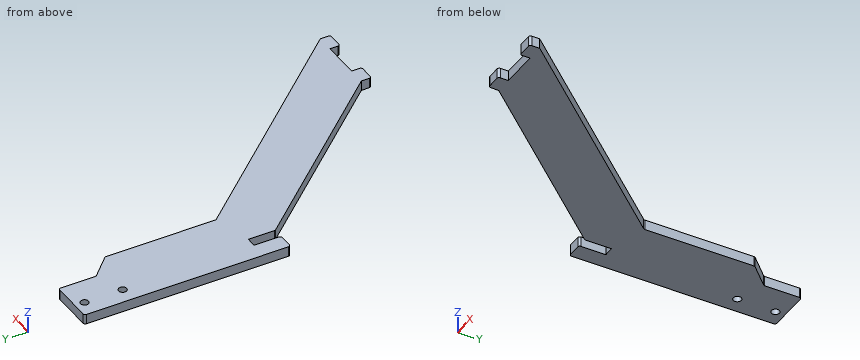
```python
from build123d import *

# Parameters (mm, degrees)
SKETCH1_R           = 1.89865
BOSS_EXTRUDE1_DEPTH = 4.7625


with BuildPart() as part:
    # Sketch1 → Boss-Extrude1 (new body)
    with BuildSketch(Plane.XY):
        with BuildLine():
            Line((-2.175, 27), (17.118365096, 27))
            ThreePointArc((17.118365096, 27), (17.825471878, 26.707106781), (18.118365096, 26))
            Line((18.118365096, 26), (18.118365096, 9.664213562))
            ThreePointArc((18.118365096, 9.664213562), (18.194485564, 9.28153013), (18.411258315, 8.957106781))
            Line((18.411258315, 8.957106781), (27.707106781, -0.338741685))
            ThreePointArc((27.707106781, -0.338741685), (27.923879533, -0.663165034), (28, -1.045848466))
            Line((28, -1.045848466), (28, -52.620004972))
            ThreePointArc((28, -52.620004972), (28.065214876, -52.975218671), (28.252353545, -53.284101936))
            Line((28.252353545, -53.284101936), (116.825, -153))
            Line((116.825, -153), (116.825, -156.7625))
            ThreePointArc((116.825, -156.7625), (116.532106781, -157.469606781), (115.825, -157.7625))
            Line((115.825, -157.7625), (109.825, -157.7625))
            ThreePointArc((109.825, -157.7625), (109.117893219, -157.469606781), (108.825, -156.7625))
            Line((108.825, -156.7625), (108.825, -153))
            Line((108.825, -153), (90.851723172, -153))
            Line((90.851723172, -153), (90.851723172, -156.7625))
            ThreePointArc((90.851723172, -156.7625), (90.558829954, -157.469606781), (89.851723172, -157.7625))
            Line((89.851723172, -157.7625), (83.851723172, -157.7625))
            ThreePointArc((83.851723172, -157.7625), (83.144616391, -157.469606781), (82.851723172, -156.7625))
            Line((82.851723172, -156.7625), (82.851723172, -153))
            Line((82.851723172, -153), (9.777353545, -70.73220419))
            ThreePointArc((9.777353545, -70.73220419), (9.590214876, -70.423320926), (9.525, -70.068107226))
            Line((9.525, -70.068107226), (9.525, -57.748102255))
            Line((9.525, -57.748102255), (4.7625, -57.748102255))
            Line((4.7625, -57.748102255), (4.7625, -69.448102255))
            ThreePointArc((4.7625, -69.448102255), (4.469606781, -70.155209036), (3.7625, -70.448102255))
            Line((3.7625, -70.448102255), (-2.175, -70.448102255))
            ThreePointArc((-2.175, -70.448102255), (-2.882106781, -70.155209036), (-3.175, -69.448102255))
            Line((-3.175, -69.448102255), (-3.175, 26))
            ThreePointArc((-3.175, 26), (-2.882106781, 26.707106781), (-2.175, 27))
        make_face()
        with Locations(Location((4.5, 22.5, 0), (0, 0, 180))):
            Circle(SKETCH1_R, mode=Mode.SUBTRACT)
        with Locations(Location((4.5, 4.5, 0), (0, 0, 180))):
            Circle(SKETCH1_R, mode=Mode.SUBTRACT)
    extrude(amount=BOSS_EXTRUDE1_DEPTH)


solid = part.part
```
Can you work these out from the model? Positions are in its coordinate system, mm. Give positions to 0.01 mm unless a question says otherwise; leave off trailing zeros. Loops run counter-clockwise (first coordinate to the right, second up) from the corner with the lowest first, then second, coordinate; pieces in that order, holes last. Notation, with made-up numbers: M -4.5,-13.75 L 39.5,-13.75 A34 ccw 39.5,20.25 Z; hole C 28.25,25 d7. An arc over 180 degrees is marked long. Use CSV: the item, a comma, the result in double quotes. Start each with the question number.
1. For P1, Ø2.5, axis at x = 103.5, z = 3, coming from the -Y side; P2, Ø1.1, axis at y = -155.5, z = 3, coming from the -X side; P3, Ø2.5, axis at y = 19, z = 3, coming from the +X side, each with a flat end and sliding along its axis, tell me the tip position at first contact or that it passes through.
2. Imagine slicing it at A-A, the plane y = 22.5. Write out the boundary of the cut face in (x, z) (1 decimal).
3. If I drill on L1, parallel to Y at x = 4.5, z = 1.25; L2, parallel to X at y = 22.5, z = 2.85 (3 decimals); L3, parallel to X at y = -1, z = 1.95 (3 decimals), over which ranges is the centre line in solid material (lowest first)?
4. Imagine slicing it at C-C, the plane y = -28.5. Write out the boundary of the cut face in (x, z) (1 decimal), plus the area to 3 significant figures.
5. Imagine slicing it at B-B, the plane z = 1.95. Count the separate pieces of the cut face and the enclosed holes in it, plus the area to 3 significant figures.
6. Imagine slicing it at D-D, the plane x = 45. Write out the boundary of the cut face in (y, z).
Response values:
1,P1,"y = -153"
1,P2,"x = 82.85"
1,P3,"x = 18.12"
2,outline,"M -3.2,0 L 2.6,0 L 2.6,4.8 L -3.2,4.8 Z; M 6.4,0 L 18.1,0 L 18.1,4.8 L 6.4,4.8 Z"
3,L1,"-70.12 to 2.6, 6.4 to 20.6, 24.4 to 27"
3,L2,"-3.175 to 2.601, 6.399 to 18.118"
3,L3,"-3.175 to 27.999"
4,outline,"M -3.2,0 L 28,0 L 28,4.8 L -3.2,4.8 Z"
4,area,"148 mm^2"
5,separate pieces,"1"
5,enclosed holes,"2"
5,area,"5,740 mm^2"
6,outline,"M -110.39,0 L -72.14,0 L -72.14,4.76 L -110.39,4.76 Z"
